For this review, take the finished solid that the model builds, in its own axes (mm). A direction names the side the tool comes from. Give positions to 0.01 mm unless a question says otherwise; leave off trailing zeros. Loops run counter-clockwise (first coordinate to the right, second up) from the corner with the lowest first, then second, coordinate; pieces in that order, holes last.
Autodesk Inventor part; units mm, degrees
ref_plane "YZ Plane" through (0, 0, 0) normal (1, 0, 0) x (0, 1, 0)
ref_plane "XZ Plane" through (0, 0, 0) normal (0, 1, 0) x (-1, 0, 0)
ref_plane "XY Plane" through (0, 0, 0) normal (0, 0, 1) x (1, 0, 0)
sketch "Sketch1" plane through (0, 0, 0) normal (0, 0, 1) x (1, 0, 0)
  circle A0 centre (0, 0) radius 8.5
  dimension "d0" = 17
extrude "Extrusion1" add sketch "Sketch1" along normal blind 5
sketch "Sketch2" plane through (0, 0, 5) normal (0, 0, 1) x (1, 0, 0)
  circle A0 centre (0, 0) radius 3.75
  circle A1 centre (0, 0) radius 8.5
  dimension "d3" = 7.5
extrude "Extrusion2" cut sketch "Sketch2" against normal blind 4
sketch "Sketch3" plane through (0, 0, 5) normal (0, 0, 1) x (1, 0, 0)
  circle A0 centre (0, 0) radius 1.75
  dimension "d6" = 3.5
extrude "Extrusion3" cut sketch "Sketch3" against normal through all
properties part number "fijador.rodamiento02"
Item 1: Tool access review of faces 4 (the flat face through (1, -2, 5)), 5 (the cylindrical face through (-3.746, 0.165, 3.028)): name each direction out of +Z, -Z, +X, -X, +Y, -Y from which nothing blocks a thin tool from reaching the whole face with its end or side.
Answer:
face 4: +Z, +X, -X, +Y, -Y
face 5: +Z
Item 2: The part is to be moulded in two halves that separate along X. For faces 1 (the cylindrical face through (4.57, -7.167, 0.493)), 2 (the cylindrical face through (1.617, -0.67, 2.535)), 3 (the flat face through (4, -2, 1)), say which applies: released by +X, released by -X, zero draft, split by the parting line, or undercut.
Answer:
face 1: split by the parting line
face 2: undercut
face 3: zero draft
Item 3: Clearance check with flat-ended pins moving along their axes: pin 1 Ø1 at (y, z) = (3, 3.5) entering from -X; pin 2 Ø4 at (x, y) = (-2.5, 5) entering from -Z; pin 3 Ø1 at (x, y) = (5, 5) entering from +Z. State where each tip first meets the part, or that it passes through.
Answer:
pin 1: stops at x = -2.8
pin 2: stops at z = 0
pin 3: stops at z = 1
Item 4: Take a section at D-D on y = 4. Give the boundary of the cut face in (x, z), and give its area (3 significant figures).
Answer:
outline: (-7.5, 0) - (7.5, 0) - (7.5, 1) - (-7.5, 1) - close
area: 15.0 mm2
Item 5: Take a section at A-A on y = 0. Give the boundary of the cut face in (x, z), and give its area (3 significant figures).
Answer:
outline: (-8.5, 0) - (-1.75, 0) - (-1.75, 5) - (-3.75, 5) - (-3.75, 1) - (-8.5, 1) - close; (1.75, 0) - (8.5, 0) - (8.5, 1) - (3.75, 1) - (3.75, 5) - (1.75, 5) - close
area: 29.5 mm2
Item 6: For L1, parallel to Y at x = 0, z = 1.7; L2, parallel to Z at x = 7, y = -4.75; L3, parallel to Y at x = -1.25, z = 4.6, list the stretches that pass through material, from the lowest coordinate up.
Answer:
L1: y = -3.75 to -1.75, 1.75 to 3.75
L2: z = 0 to 1
L3: y = -3.54 to -1.22, 1.22 to 3.54
Item 7: Take a section at C-C on z = 2.6. Give the boundary of the cut face in (x, y), and give its area (3 significant figures).
Answer:
outline: circle Ø7.5 at (0, 0); hole circle Ø3.5 at (0, 0)
area: 34.6 mm2
